Work out the finished part from the listing and answer in its coordinate system (mm). A direction names the side the tool comes from. Round coordinates to 2 decimals unless told otherwise and drop trailing zeros. Write each loop counter-clockwise with the first axis right and the second up, starting at its lowest first coordinate (ties: lowest second). Pieces come first, ordered by that corner, then holes. Notation, with made-up numbers: M 30.5,-7.75 L 63.5,-7.75 A7 cw 63.5,3.25 Z; hole C 60,-3.75 d9. An arc over 180 degrees is marked long. One line per item, written item: value. Start each with the question number.
Q1. Find section A-A (y = 9). Write down the section's boundary in (x, z).
Q2. A tool of negligible diameter and unlimited length cuts with its end or side. For faces 1 (the cylindrical face through (9.27, 7.85, 4.52)), 2 (the cylindrical face through (24.1, 14.14, 3.04)), 3 (the flat face through (20, 6, 3)), from which of +Z, -Z, +X, -X, +Y, -Y can it reach the whole face along a straight path? Write none if from no direction.
Q3. The mould has two halves that part along X. Classify faces 4 (the cylindrical face through (20.5, 0.5, 5.1)), 5 (the flat face through (12, 8, 0)), 6 (the flat face through (25, 6, 3)): released by +X, released by -X, zero draft, split by the parting line, or undercut.
Q4. Find section C-C (z = 5). Write down the section's boundary in (x, y).
Q5. Consider probe 1 along X at (y, z) = (9, 2); probe 2 along X at (y, z) = (1.5, 3); probe 3 along Y at (x, z) = (18.5, 0.85). Determine where each line is inside the solid, lowest interval first.
Q6. Given pin 1 Ø2.5 at (x, z) = (4, 2.5) entering from -Y; pin 2 Ø1.8 at (x, y) = (7.5, 9.5) entering from +Z; pin 3 Ø1.5 at (x, z) = (21, 2.5) entering from -Y, each flat-ended and moving along its own axis, determine where each tip first touches the part or whether it passes through.
Q7. Find section D-D (y = 3.5). Write down the section's boundary in (x, z), and give its area (3 significant figures).
Q8. Find section B-B (x = 18.5). Write down the section's boundary in (y, z), and give its area (3 significant figures).
from build123d import *

# Parameters (mm, degrees)
SKETCH_1_W          = 25
SKETCH_1_H          = 15
SKETCH_1_R          = 1.55
EXTRUDE_1_DEPTH     = 6
SKETCH_3_R          = 1.5
CUT_EXTRUDE_1_DEPTH = 6
CUT_EXTRUDE_2_DEPTH = 30.765752132
FILLET_1_R          = 3
SKETCH_5_R          = 3
CUT_EXTRUDE_3_DEPTH = 3


with BuildPart() as part:
    # ｽｹｯﾁ1 → ﾎﾞｽ - 押し出し1 (new body)
    with BuildSketch(Plane.XY):
        with Locations((12.5, 7.5)):
            Rectangle(SKETCH_1_W, SKETCH_1_H)
        with Locations((6.5, 9)):
            Circle(SKETCH_1_R, mode=Mode.SUBTRACT)
        with Locations(Location((18.5, 9, 0), (0, 0, 180))):
            Circle(SKETCH_1_R, mode=Mode.SUBTRACT)
    extrude(amount=EXTRUDE_1_DEPTH)

    # ｽｹｯﾁ3 → ｶｯﾄ - 押し出し1 (cut)
    with BuildSketch(Plane.XZ):
        with Locations(Location((4.5, 3, 0), (0, 0, 270))):
            Circle(SKETCH_3_R)
        with Locations(Location((20.5, 3, 0), (0, 0, 90))):
            Circle(SKETCH_3_R)
    extrude(amount=-CUT_EXTRUDE_1_DEPTH, mode=Mode.SUBTRACT)

    # ｽｹｯﾁ4 → ｶｯﾄ - 押し出し2 (cut, through all)
    with BuildSketch(Plane.XY.offset(6)):
        with BuildLine():
            Line((3.177124344, 0), (5.822875656, 0))
            ThreePointArc((5.822875656, 0), (4.5, 0.5), (3.177124344, 0))
        make_face()
        with BuildLine():
            Line((21.822875656, 0), (19.177124344, 0))
            ThreePointArc((19.177124344, 0), (20.5, 0.5), (21.822875656, 0))
        make_face()
    extrude(amount=-CUT_EXTRUDE_2_DEPTH, mode=Mode.SUBTRACT)

    # ﾌｨﾚｯﾄ1
    fillet_1_edges = [part.edges().sort_by_distance(p)[0] for p in [
        (0, 15, 3),
        (25, 15, 3),
    ]]
    fillet(fillet_1_edges, radius=FILLET_1_R)

    # ｽｹｯﾁ5 → ｶｯﾄ - 押し出し3 (cut)
    with BuildSketch(Plane.XY.offset(6)):
        with Locations((6.5, 9)):
            Circle(SKETCH_5_R)
        with Locations((18.5, 9)):
            Circle(SKETCH_5_R)
    extrude(amount=-CUT_EXTRUDE_3_DEPTH, mode=Mode.SUBTRACT)


solid = part.part
The answers:
1. outline: M 0,0 L 4.95,0 L 4.95,3 L 3.5,3 L 3.5,6 L 0,6 Z; M 8.05,0 L 16.95,0 L 16.95,3 L 15.5,3 L 15.5,6 L 9.5,6 L 9.5,3 L 8.05,3 Z; M 20.05,0 L 25,0 L 25,6 L 21.5,6 L 21.5,3 L 20.05,3 Z
2. face 1: +Z
2. face 2: +Z, -Z, +X, +Y
2. face 3: -Y
3. face 4: undercut
3. face 5: zero draft
3. face 6: released by +X
4. outline: M 0,0 L 3.18,0 A2 cw 5.82,0 L 19.18,0 A2 cw 21.82,0 L 25,0 L 25,12 A3 ccw 22,15 L 3,15 A3 ccw 0,12 Z; hole C 6.5,9 d6; hole C 18.5,9 d6
5. probe 1: 0 to 4.95, 8.05 to 16.95, 20.05 to 25
5. probe 2: 0 to 3, 6 to 19, 22 to 25
5. probe 3: 0 to 7.45, 10.55 to 15
6. pin 1: y = 0
6. pin 2: z = 3
6. pin 3: y = 6
7. outline: M 0,0 L 25,0 L 25,6 L 0,6 Z; hole C 4.5,3 d3; hole C 20.5,3 d3
7. area: 136 mm2
8. outline: M 0,0 L 7.45,0 L 7.45,3 L 6,3 L 6,6 L 0,6 Z; M 10.55,0 L 15,0 L 15,6 L 12,6 L 12,3 L 10.55,3 Z
8. area: 62.7 mm2
